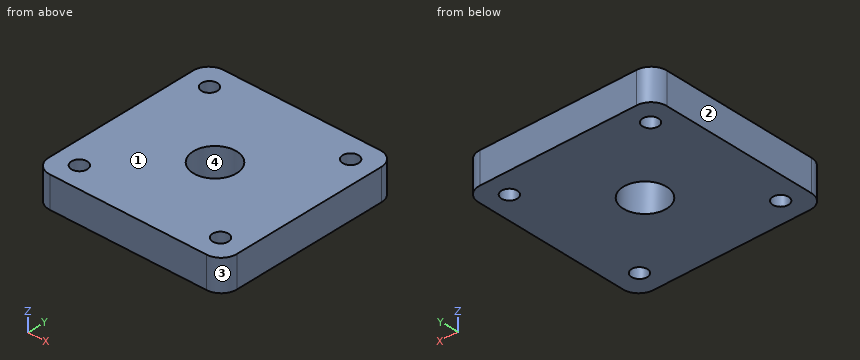
from build123d import *

# Parameters (mm, degrees)
SKETCH1_R           = 8.73125
SKETCH1_R_2         = 3.1877
BOSS_EXTRUDE1_DEPTH = 12.7
SCALE1_SCALE        = 0.66


with BuildPart() as part:
    # Sketch1 → Boss-Extrude1 (new body)
    with BuildSketch(Plane.XY):
        with BuildLine():
            Line((-31.75, 38.1), (31.75, 38.1))
            ThreePointArc((31.75, 38.1), (36.240128061, 36.240128061), (38.1, 31.75))
            Line((38.1, 31.75), (38.1, -31.75))
            ThreePointArc((38.1, -31.75), (36.240128061, -36.240128061), (31.75, -38.1))
            Line((31.75, -38.1), (-31.75, -38.1))
            ThreePointArc((-31.75, -38.1), (-36.240128061, -36.240128061), (-38.1, -31.75))
            Line((-38.1, -31.75), (-38.1, 31.75))
            ThreePointArc((-38.1, 31.75), (-36.240128061, 36.240128061), (-31.75, 38.1))
        make_face()
        Circle(SKETCH1_R, mode=Mode.SUBTRACT)
        with Locations((-28.575, 28.575)):
            Circle(SKETCH1_R_2, mode=Mode.SUBTRACT)
        with Locations((28.575, 28.575)):
            Circle(SKETCH1_R_2, mode=Mode.SUBTRACT)
        with Locations((28.575, -28.575)):
            Circle(SKETCH1_R_2, mode=Mode.SUBTRACT)
        with Locations((-28.575, -28.575)):
            Circle(SKETCH1_R_2, mode=Mode.SUBTRACT)
    extrude(amount=BOSS_EXTRUDE1_DEPTH)


with BuildPart() as part_1:
    # Scale1: scaled about (0, 0, 6.35)
    add(part.part.scale(SCALE1_SCALE).moved(Location((0, 0, 2.159))))


solid = part_1.part
Read the model definition and answer for the solid it produces. Units are mm, in the model's axes. Face numbers are marked on the shaded views. Give positions to 0.01 mm unless a question says otherwise; leave off trailing zeros. Write each loop counter-clockwise with the first axis right and the second up, starting at its lowest first coordinate (ties: lowest second). Pieces come first, ordered by that corner, then holes. Notation, with made-up numbers: (-6.75, 42.5) - (2.25, 42.5) arc R23 cw to (2.25, 74.5) - close; hole circle Ø9 at (-33, 79.5). An arc over 180 degrees is marked (long way). Return JSON: item names as keys, results as strings.
Q1. Consider line 1 along Y through (x, z) = (-19, 8.5); line 2 along X through (y, z) = (-17, 4.5). Determine where each line is inside the solid, lowest interval first. Write a range as [from, to].
Reply:
{"line 1": "[-25.15, -20.96], [-16.76, 16.76], [20.96, 25.15]", "line 2": "[-25.15, -19.84], [-17.88, 17.88], [19.84, 25.15]"}
Q2. A cutting plane is placed at D-D, the plane x = -17.5. Determine the outline of the cut face in (y, z).
Reply:
{"outline": "(-25.15, 2.16) - (-20.47, 2.16) - (-20.47, 10.54) - (-25.15, 10.54) - close; (-17.25, 2.16) - (17.25, 2.16) - (17.25, 10.54) - (-17.25, 10.54) - close; (20.47, 2.16) - (25.15, 2.16) - (25.15, 10.54) - (20.47, 10.54) - close"}
Q3. Given P1, Ø3.5, axis at x = 18.86, y = 18.86, coming from the -Z side, flat-ended and moving along its own axis, determine where the tip first touches the part or whether it passes through.
Reply:
{"P1": "through"}
Q4. For a pull along X with two mould halves and no side action, classify the marked faces 1, 2, 3 and 4 as released by +X, released by -X, zero draft, split by the parting line, or undercut.
Reply:
{"face 1": "zero draft", "face 2": "released by -X", "face 3": "released by +X", "face 4": "undercut"}
Q5. A cutting plane is placed at C-C, the plane y = 20. Determine the outline of the cut face in (x, z).
Reply:
{"outline": "(-25.15, 2.16) - (-20.63, 2.16) - (-20.63, 10.54) - (-25.15, 10.54) - close; (-17.09, 2.16) - (17.09, 2.16) - (17.09, 10.54) - (-17.09, 10.54) - close; (20.63, 2.16) - (25.15, 2.16) - (25.15, 10.54) - (20.63, 10.54) - close"}
Q6. A cutting plane is placed at A-A, the plane x = 0. Determine the outline of the cut face in (y, z), and give its area (3 significant figures).
Reply:
{"outline": "(-25.15, 2.16) - (-5.76, 2.16) - (-5.76, 10.54) - (-25.15, 10.54) - close; (5.76, 2.16) - (25.15, 2.16) - (25.15, 10.54) - (5.76, 10.54) - close", "area": "325 mm²"}
